The model under review builds one solid part; all positions refer to its coordinate system, in mm. A direction names the side the tool comes from. Round coordinates to 2 decimals unless told otherwise and drop trailing zeros. Write each loop counter-clockwise with the first axis right and the second up, starting at its lowest first coordinate (ties: lowest second). Pieces come first, ordered by that corner, then holes. Notation, with made-up numbers: (-38.75, 9.5) - (17.25, 9.5) arc R10 ccw to (17.25, 19.5) - close; hole circle Ø3 at (30.25, 76). An arc over 180 degrees is marked (long way). Write each question's results on one line, items separated by ' | '.
```python
from build123d import *

# Parameters (mm, degrees)
F0_W      = 20
F0_H      = 660
F0_H_2    = 20
F1_DEPTH  = 20
F2_DEPTH  = 580
F3_W      = 20
F3_H      = 20
F4_DEPTH  = 660
F5_W      = 20
F5_H      = 20
F6_DEPTH  = 560
F7_W      = 20
F7_H      = 20
F8_DEPTH  = 560
F9_W      = 20
F9_H      = 20
F10_DEPTH = 660


# Not quite as in the source:
# - a feature names something its author has since deleted; it is built from what else it names


with BuildPart() as f1:
    # F0 (on Top) → F1 (new body)
    with BuildSketch(Plane.XY):
        Polygon((250.936165452, 480.5163520575), (-329.063834548, 480.5163520575), (-329.063834548, 460.5163520575), (230.936165452, 460.5163520575), (230.936165452, -199.4836479425), (-329.063834548, -199.4836479425), (-329.063834548, -219.4836479425), (250.936165452, -219.4836479425), align=None)
        with Locations((-339.063834548, 130.5163520575)):
            Rectangle(F0_W, F0_H)
        with Locations((-339.063834548, 470.5163520575)):
            Rectangle(F0_W, F0_H_2)
        with Locations((-339.063834548, -209.4836479425)):
            Rectangle(F0_W, F0_H_2)
    extrude(amount=F1_DEPTH)

    # F0 (on Top) → F2 (join)
    with BuildSketch(Plane.XY):
        with Locations((-339.063834548, 470.5163520575)):
            Rectangle(F0_W, F0_H_2)
        with Locations((-339.063834548, -209.4836479425)):
            Rectangle(F0_W, F0_H_2)
    extrude(amount=F2_DEPTH)

    # F3 (on face) → F4 (join)
    with BuildSketch(Plane(origin=(0, -199.4836479425, 0), x_dir=(-1, 0, 0), z_dir=(0, 1, 0))):
        with Locations((339.063834548, 570)):
            Rectangle(F3_W, F3_H)
    extrude(amount=F4_DEPTH)

    # F5 (on face) → F6 (join)
    with BuildSketch(Plane.YZ.offset(-329.063834548)):
        with Locations((-209.4836479425, 570)):
            Rectangle(F5_W, F5_H)
        with Locations((470.5163520575, 570)):
            Rectangle(F5_W, F5_H)
    extrude(amount=F6_DEPTH)

    # F7 (on face) → F8 (join)
    with BuildSketch(Plane.XY.offset(20)):
        with Locations((240.936165452, 470.5163520575)):
            Rectangle(F7_W, F7_H)
        with Locations((240.936165452, -209.4836479425)):
            Rectangle(F7_W, F7_H)
    extrude(amount=F8_DEPTH)

    # F9 (on face) → F10 (join)
    with BuildSketch(Plane.XZ.offset(-460.5163520575)):
        with Locations((240.936165452, 570)):
            Rectangle(F9_W, F9_H)
    extrude(amount=F10_DEPTH)


solid = f1.part
```
Q1. We need section B-B (x = -159.5). State the section outline as (y, z) points, plus the area to 3 significant figures.
Evaluation:
outline: (-219.48, 0) - (-199.48, 0) - (-199.48, 20) - (-219.48, 20) - close; (-219.48, 560) - (-199.48, 560) - (-199.48, 580) - (-219.48, 580) - close; (460.52, 0) - (480.52, 0) - (480.52, 20) - (460.52, 20) - close; (460.52, 560) - (480.52, 560) - (480.52, 580) - (460.52, 580) - close | area: 1,600 mm^2
Q2. We need section A-A (z = 170.5). State the section outline as (x, y) points.
Evaluation:
outline: (-349.06, -219.48) - (-329.06, -219.48) - (-329.06, -199.48) - (-349.06, -199.48) - close; (-349.06, 460.52) - (-329.06, 460.52) - (-329.06, 480.52) - (-349.06, 480.52) - close; (230.94, -219.48) - (250.94, -219.48) - (250.94, -199.48) - (230.94, -199.48) - close; (230.94, 460.52) - (250.94, 460.52) - (250.94, 480.52) - (230.94, 480.52) - close
Q3. Insertion check: P1, Ø16, axis at x = -79, y = 473.5, coming from the -Z side. The pin has a flat end and moves straight along its axis. Give the tip position at first contact, or say it passes through.
Evaluation:
P1: stops at z = 0
Q4. The part is to be moulded in two halves that separate along Y. For faces 6 (the flat face through (-339, 132, 580)), 7 (the flat face through (241, 460.516, 286)), 8 (the flat face through (-339, 126, 560)), 9 (the flat face through (-50, -219.484, 9)), say which applies: released by +Y, released by -Y, zero draft, split by the parting line, or undercut.
Evaluation:
face 6: zero draft | face 7: undercut | face 8: undercut | face 9: released by -Y
Q5. Tool access review of faces 1 (the flat face through (-329.064, -210, 286)), 2 (the flat face through (-73, 480.516, 568)), 3 (the flat face through (241, 135, 20)), 4 (the flat face through (230.936, 135, 10)), 5 (the flat face through (-349.064, 129, 9)): name each direction out of +Z, -Z, +X, -X, +Y, -Y from which nothing blocks a thin tool from reaching the whole face with its end or side.
Evaluation:
face 1: +Y, -Y | face 2: +Z, -Z, +X, -X, +Y | face 3: +X, -X | face 4: +Z, -Z | face 5: +Z, -Z, -X, +Y, -Y
